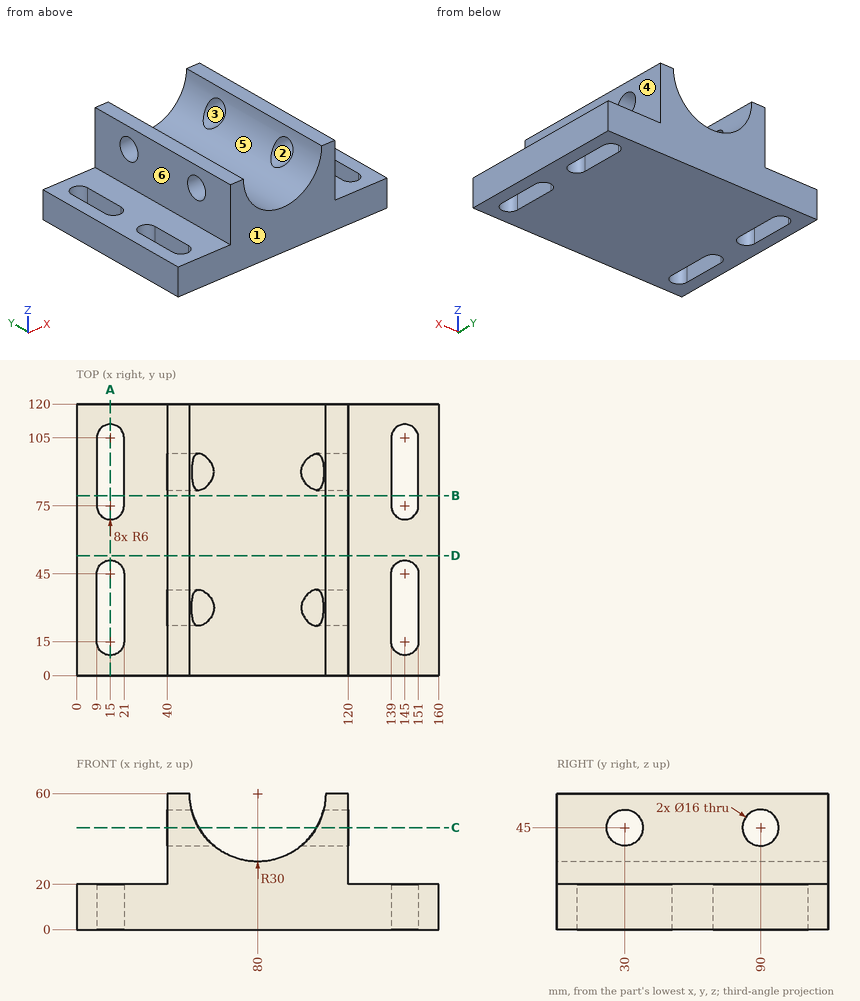
Answer from the drawing. Dimensions are ordinates in mm from the lowest x, y and z of the part. A direction names the side the tool comes from. Give positions to 0.01 mm unless a question says otherwise; leave off trailing zeros. Order: outer loops, then holes, each group sorted by start corner. A loop starts at its lowest first (then second) coordinate and runs counter-clockwise, first axis right, second up.
(1) Find section B-B (y = 79.5). Give the vertices of the cut face in (x, z).
(2) Find section D-D (y = 53). Give the vertices of the cut face in (x, z), plus the area to 3 significant figures.
(3) Find section C-C (z = 45). Give the vertices of the cut face in (x, y), plus the area to 3 significant figures.
(4) For a pull along Y with two mould halves and no side action, classify the marked faces 1, 2, 3 and 4 as released by +Y, released by -Y, zero draft, split by the parting line, or undercut.
(5) For the marked faces 5 and 6, determine the directions among +Z, -Z, +X, -X, +Y, -Y from which every point of the face is accessible in a straight line to the end or side of a thin tool.
(6) Find section A-A (x = 15). Give the vertices of the cut face in (y, z), plus the area to 3 significant figures.
(7) Given pin 1 (13 mm diameter, centred on y = 90, z = 45, fed in from +X); pin 2 (12 mm diameter, centred on x = 18.5, y = 74, fed in from +Z); pin 3 (3 mm diameter, centred on y = 69.5, z = 23, fed in from -X); pin 4 (18.5 mm diameter, centred on y = 30, z = 45, fed in from +X), each flat-ended and moving along its own axis, determine where each tip first touches the part or whether it passes through.
(8) Straight lines are drawn through the part: L1, parallel to X at y = 83.5, z = 13; L2, parallel to Y at x = 115.75, z = 45; L3, parallel to Z at x = 49, y = 30. For each, find the intervals that lie inside material, in ascending order.
Result sheet:
1. outline: (0, 0) - (9, 0) - (9, 20) - (0, 20) - close; (21, 0) - (139, 0) - (139, 20) - (120, 20) - (120, 60) - (110, 60) arc R30 cw to (50, 60) - (40, 60) - (40, 20) - (21, 20) - close; (151, 0) - (160, 0) - (160, 20) - (151, 20) - close
2. outline: (0, 0) - (160, 0) - (160, 20) - (120, 20) - (120, 60) - (110, 60) arc R30 cw to (50, 60) - (40, 60) - (40, 20) - (0, 20) - close
2. area: 4,990 mm2
3. outline: (40, 0) - (54.02, 0) - (54.02, 22) - (40, 22) - close; (40, 38) - (54.02, 38) - (54.02, 82) - (40, 82) - close; (40, 98) - (54.02, 98) - (54.02, 120) - (40, 120) - close; (105.98, 0) - (120, 0) - (120, 22) - (105.98, 22) - close; (105.98, 38) - (120, 38) - (120, 82) - (105.98, 82) - close; (105.98, 98) - (120, 98) - (120, 120) - (105.98, 120) - close
3. area: 2,470 mm2
4. face 1: released by -Y
4. face 2: undercut
4. face 3: undercut
4. face 4: zero draft
5. face 5: +Z, +Y, -Y
5. face 6: +Z, -X, +Y, -Y
6. outline: (0, 0) - (9, 0) - (9, 20) - (0, 20) - close; (51, 0) - (69, 0) - (69, 20) - (51, 20) - close; (111, 0) - (120, 0) - (120, 20) - (111, 20) - close
6. area: 720 mm2
7. pin 1: passes through
7. pin 2: stops at z = 20
7. pin 3: stops at x = 40
7. pin 4: stops at x = 120
8. L1: x = 0 to 9, 21 to 139, 151 to 160
8. L2: y = 0 to 22, 38 to 82, 98 to 120
8. L3: z = 0 to 37, 53 to 60
